Could you check a few things on this model? Use its own coordinates, in mm. A direction names the side the tool comes from. Coordinates: 2 decimals unless noted, no trailing zeros. Order: outer loops, then holes, each group sorted by start corner. A loop starts at its lowest first (then second) coordinate and runs counter-clockwise, first axis right, second up. Notation, with made-up numbers: (-39.5, 89) - (18.5, 89) arc R8 cw to (18.5, 103) - close; hole circle Ø7 at (50.25, 79.5). An arc over 180 degrees is marked (long way). Answer as a JSON object with one key per item and string values. Group by question number.
(1) Imagine slicing it at D-D, the plane x = 0. Write out the boundary of the cut face in (y, z) (3 decimals), and give its area (3 significant figures).
(2) We'd pull the mould along Y, two halves only. Please class faces 1 (the flat face through (-9, 4.657, 0)), 2 (the flat face through (-9, 3.657, 0)), 3 (the flat face through (-12.7, 9.4, 0)), 4 (the flat face through (-9, 8.929, 0)): pulls with the +Y half, pulls with the -Y half, needs draft (parallel to the pull), parting line crosses it, or undercut.
(3) Imagine slicing it at B-B, the plane z = 1.5. Write out the boundary of the cut face in (x, y).
(4) Imagine slicing it at A-A, the plane x = -11. Write out the boundary of the cut face in (y, z).
(5) Imagine slicing it at C-C, the plane y = 11.75. Write out the boundary of the cut face in (x, z) (3 decimals), and give its area (3 significant figures).
(6) Please list where these lines run through material, in increasing order: probe 1 along X at (y, z) = (11.9, 0); probe 2 along Z at (x, y) = (0, 10.7) (3 decimals); probe 3 along Y at (x, z) = (0.25, -0.75).
(7) Which directions (+Z, -Z, +X, -X, +Y, -Y) give clear straight access to the entire face, cutting with the end or side of a thin tool? Please do faces 5 (the flat face through (0, 9.7, 0)), 6 (the flat face through (-9, 9.929, 0)), 7 (the flat face through (-9, 4, -1.713)), 8 (the flat face through (-9.5, 9.4, 1.787)).
(8) Will these pins go through, and if not, where does the flat tip stop? P1, Ø1.8, axis at x = -11, z = -0.5, coming from the +Y side; P2, Ø4, axis at x = -8.5, y = 10.5, coming from the -Z side; P3, Ø0.7, axis at x = 0, z = 0, coming from the +Y side.
from build123d import *

# Parameters (mm, degrees)
SKETCH1_W           = 12.7
SKETCH1_H           = 6.35
BOSS_EXTRUDE1_DEPTH = 12.7
SKETCH2_R           = 1.190625
CUT_EXTRUDE1_DEPTH  = 3
SKETCH3_W           = 3.5
SKETCH3_H           = 1
BOSS_EXTRUDE2_DEPTH = 6.35


with BuildPart() as part:
    # Sketch1 → Boss-Extrude1 (new body)
    with BuildSketch(Plane(origin=(0, 0, 0), x_dir=(1, 0, 0), z_dir=(0, 1, 0))):
        Rectangle(SKETCH1_W, SKETCH1_H)
    extrude(amount=BOSS_EXTRUDE1_DEPTH)

    # Sketch2 → Cut-Extrude1 (cut)
    with BuildSketch(Plane(origin=(0, 12.7, 0), x_dir=(1, 0, 0), z_dir=(0, 1, 0))):
        Circle(SKETCH2_R)
    extrude(amount=-CUT_EXTRUDE1_DEPTH, mode=Mode.SUBTRACT)

    # Sketch3 → Boss-Extrude2 (add)
    with BuildSketch(Plane.ZY.offset(6.35)):
        with Locations((0.037458048, 4.156500498)):
            Rectangle(SKETCH3_W, SKETCH3_H)
        with Locations((0.037458048, 9.428549286)):
            Rectangle(SKETCH3_W, SKETCH3_H)
    extrude(amount=BOSS_EXTRUDE2_DEPTH)


solid = part.part
Result set:
{
 "1": {"outline": "(0, -3.175) - (12.7, -3.175) - (12.7, -1.191) - (9.7, -1.191) - (9.7, 1.191) - (12.7, 1.191) - (12.7, 3.175) - (0, 3.175) - close", "area": "73.5 mm^2"},
 "2": {"face 1": "undercut", "face 2": "pulls with the -Y half", "face 3": "needs draft", "face 4": "undercut"},
 "3": {"outline": "(-12.7, 3.66) - (-6.35, 3.66) - (-6.35, 0) - (6.35, 0) - (6.35, 12.7) - (-6.35, 12.7) - (-6.35, 9.93) - (-12.7, 9.93) - (-12.7, 8.93) - (-6.35, 8.93) - (-6.35, 4.66) - (-12.7, 4.66) - close"},
 "4": {"outline": "(3.66, -1.71) - (4.66, -1.71) - (4.66, 1.79) - (3.66, 1.79) - close; (8.93, -1.71) - (9.93, -1.71) - (9.93, 1.79) - (8.93, 1.79) - close"},
 "5": {"outline": "(-6.35, -3.175) - (6.35, -3.175) - (6.35, 3.175) - (-6.35, 3.175) - close; hole circle Ø2.381 at (0, 0)", "area": "76.2 mm^2"},
 "6": {"probe 1": "x = -6.35 to -1.19, 1.19 to 6.35", "probe 2": "z = -3.175 to -1.191, 1.191 to 3.175", "probe 3": "y = 0 to 9.7"},
 "7": {"face 5": "+Y", "face 6": "+Z, -Z, -X, +Y", "face 7": "-Z, -X, +Y, -Y", "face 8": "+Z, -X, +Y, -Y"},
 "8": {"P1": "stops at y = 9.93", "P2": "stops at z = -1.71", "P3": "stops at y = 9.7"}
}
